Geometry check sheet. Reference: the model listing, model coordinates, mm. Coordinates: 2 decimals unless noted, no trailing zeros. Write each loop counter-clockwise with the first axis right and the second up, starting at its lowest first coordinate (ties: lowest second). Pieces come first, ordered by that corner, then holes.
from build123d import *

# Parameters (mm, degrees)
SKETCH1_W                     = 735.584
SKETCH1_H                     = 38.1
WOOD_BLOCK_DEPTH              = 19.05
SKETCH2_R                     = 7.9756
INNER_BORE_DEPTH              = 737.816349952
SKETCH3_R                     = 6.3881
MOUTHPIECE_THROUGH_HOLE_DEPTH = 737.816349952
SKETCH5_R                     = 8.128
COUNTERBORE_DEPTH             = 5.5499
SKETCH4_OUTSIDE_W             = 187.464
SKETCH4_OUTSIDE_H             = 168.414
SKETCH4_OUTSIDE_R             = 14.2875
OUTER_DIAMETER_DEPTH          = 737.816350054


with BuildPart() as part:
    # Sketch1 → wood block (new body)
    with BuildSketch(Plane(origin=(0, 0, 0), x_dir=(1, 0, 0), z_dir=(0, 1, 0))):
        with Locations((367.792, 19.05)):
            Rectangle(SKETCH1_W, SKETCH1_H)
    extrude(amount=WOOD_BLOCK_DEPTH)

    # Sketch2 → inner bore (cut, through all)
    with BuildSketch(Plane(origin=(735.584, 0, 0), x_dir=(0, 0, -1), z_dir=(1, 0, 0))):
        with Locations((19.05, 19.05)):
            Circle(SKETCH2_R)
    extrude(amount=-INNER_BORE_DEPTH, mode=Mode.SUBTRACT)

    # Sketch3 → mouthpiece through hole (cut, through all)
    with BuildSketch(Plane(origin=(0, 0, 0), x_dir=(1, 0, 0), z_dir=(0, 1, 0))):
        with Locations(Location((22.225, 19.05, 0), (0, 0, 90))):
            Circle(SKETCH3_R)
    extrude(amount=MOUTHPIECE_THROUGH_HOLE_DEPTH, mode=Mode.SUBTRACT)

    # Sketch5 → counterbore (cut)
    with BuildSketch(Plane.XZ):
        with Locations(Location((22.225, -19.05, 0), (0, 0, 270))):
            Circle(SKETCH5_R)
    extrude(amount=-COUNTERBORE_DEPTH, mode=Mode.SUBTRACT)

    # Sketch4 outside → outer diameter (cut, through all)
    with BuildSketch(Plane.ZY):
        with Locations((-19.05, 9.525)):
            Rectangle(SKETCH4_OUTSIDE_W, SKETCH4_OUTSIDE_H)
        with Locations((-19.05, 19.05)):
            Circle(SKETCH4_OUTSIDE_R, mode=Mode.SUBTRACT)
    extrude(amount=-OUTER_DIAMETER_DEPTH, mode=Mode.SUBTRACT)


solid = part.part
1. Thickness scan on line 1 along Z through (x, y) = (639.5, 18.25); line 2 along X through (y, z) = (10, -19.05); line 3 along Z through (x, y) = (101.5, 15.75). Record the ranges inside material, lowest first.
Computed values:
line 1: z = -33.32 to -26.99, -11.11 to -4.78
line 2: x = 0 to 15.84, 28.61 to 735.58
line 3: z = -32.95 to -26.31, -11.79 to -5.15
2. Gauge pin test, flat ends, axial feed: pin 1 Ø1.9 at (x, z) = (16, -21) entering from -Y; pin 2 Ø1.5 at (x, y) = (404, 14.5) entering from -Z; pin 3 Ø10 at (x, z) = (22.225, -19.05) entering from -Y; pin 4 Ø5 at (x, y) = (397.5, 9) entering from -Z. Record the tip position at first contact, or that the pin passes through.
Computed values:
pin 1: stops at y = 5.55
pin 2: stops at z = -32.82
pin 3: passes through
pin 4: stops at z = -31.18
3. Sectioned sample at A-A, the plane z = -19.05. Record the boundary of the cut face in (x, y).
Computed values:
outline: (0, 4.76) - (14.1, 4.76) - (14.1, 5.55) - (15.84, 5.55) - (15.84, 11.07) - (0, 11.07) - close; (28.61, 5.55) - (30.35, 5.55) - (30.35, 4.76) - (735.58, 4.76) - (735.58, 11.07) - (28.61, 11.07) - close
4. Draft check along Z on faces 1 (the cylindrical face through (362.643, 4.766, -19.364)), 2 (the flat face through (735.584, 10, -19)), 3 (the cylindrical face through (372.941, 11.076, -18.875)). Enter one of: released by +Z, released by -Z, zero draft, split by the parting line, or undercut.
Computed values:
face 1: split by the parting line
face 2: zero draft
face 3: undercut
